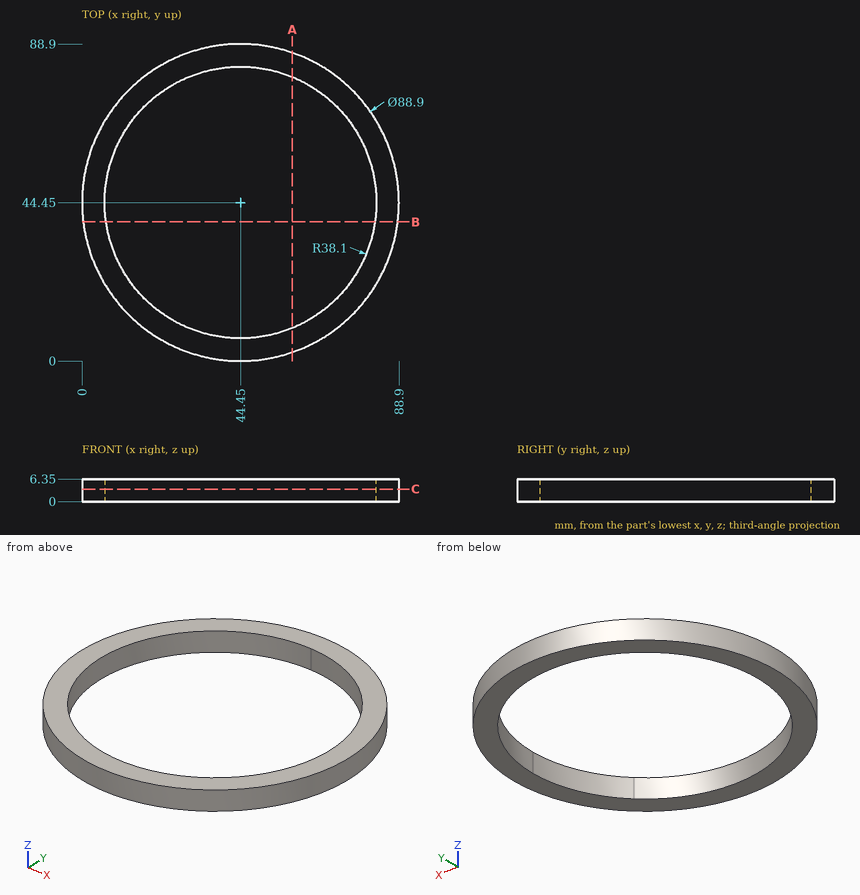
Check sheet for the drawn part. Datum: minimum x, y, z corner. Units: mm. Give positions to 0.01 mm unless a question says otherwise; leave off trailing zeros. Write each loop counter-clockwise with the first axis right and the second up, starting at its lowest first coordinate (ties: lowest second). Pieces come first, ordered by that corner, then holes.
(1) Cross-section at A-A (x = 59). Enter the section's corners in (y, z).
(2) Cross-section at C-C (z = 3.5). Enter the section's corners in (x, y), plus the area to 3 significant figures.
(3) Gauge pin test, flat ends, axial feed: pin 1 (3 mm diameter, centred on y = 19, z = 3.5, fed in from +X); pin 2 (5 mm diameter, centred on x = 76, y = 23.5, fed in from +Z); pin 3 (3 mm diameter, centred on x = 47.5, z = 5.5, fed in from +Y); pin 4 (1 mm diameter, centred on y = 50.5, z = 2, fed in from -X). Record the tip position at first contact, or that the pin passes through.
(4) Material ranges on line 1 (Y direction, x = 43.5, z = 2.25); line 2 (X direction, y = 57.5, z = 1.5); line 3 (Y direction, x = 52, z = 2), recorded low to high.
(5) Cross-section at B-B (y = 39). Enter the section's corners in (x, z).
Worked out:
1. outline: (2.45, 0) - (9.24, 0) - (9.24, 6.35) - (2.45, 6.35) - close; (79.66, 0) - (86.45, 0) - (86.45, 6.35) - (79.66, 6.35) - close
2. outline: circle Ø88.9 at (44.45, 44.45); hole (17.51, 17.51) arc R38.1 ccw to (71.39, 17.51) arc R38.1 ccw to (82.55, 44.45) arc R38.1 ccw to (44.45, 82.55) arc R38.1 ccw to start
2. area: 1,650 mm2
3. pin 1: stops at x = 81.9
3. pin 2: stops at z = 6.35
3. pin 3: stops at y = 88.87
3. pin 4: stops at x = 0.35
4. line 1: y = 0.01 to 6.36, 82.54 to 88.89
4. line 2: x = 1.96 to 8.65, 80.25 to 86.94
4. line 3: y = 0.65 to 7.11, 81.79 to 88.25
5. outline: (0.34, 0) - (6.74, 0) - (6.74, 6.35) - (0.34, 6.35) - close; (82.16, 0) - (88.56, 0) - (88.56, 6.35) - (82.16, 6.35) - close
